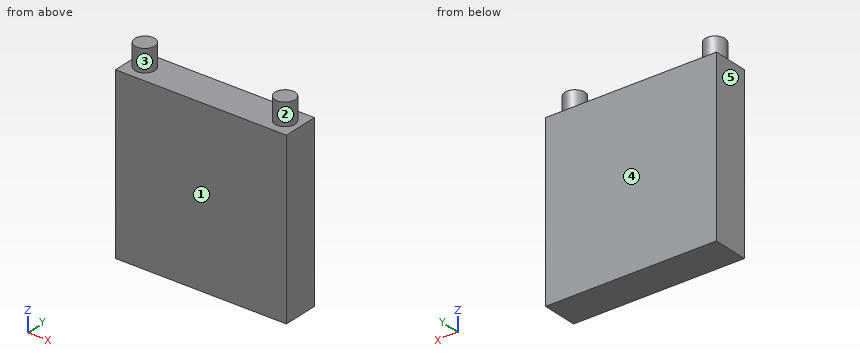
```python
from build123d import *

# Parameters (mm, degrees)
SKETCH_1_W      = 20
SKETCH_1_H      = 20
EXTRUDE_1_DEPTH = 4.2
SKETCH_2_R      = 1.173131764
EXTRUDE_2_DEPTH = 12.6


with BuildPart() as part:
    # 草图1 → 凸台-拉伸1 (new body)
    with BuildSketch(Plane(origin=(0, 0, 0), x_dir=(1, 0, 0), z_dir=(0, 1, 0))):
        Rectangle(SKETCH_1_W, SKETCH_1_H)
    extrude(amount=EXTRUDE_1_DEPTH)

    # 草图2 → 凸台-拉伸2 (add)
    with BuildSketch(Plane.XY):
        with Locations((-8.2, 2.1)):
            Circle(SKETCH_2_R)
        with Locations((8.2, 2.1)):
            Circle(SKETCH_2_R)
    extrude(amount=EXTRUDE_2_DEPTH)


solid = part.part
```
For this review, take the finished solid that the model builds, in its own axes (mm). Face numbers are marked on the shaded views. A direction names the side the tool comes from. Coordinates: 2 decimals unless noted, no trailing zeros. Write each loop counter-clockwise with the first axis right and the second up, starting at its lowest first coordinate (ties: lowest second). Pieces come first, ordered by that corner, then holes. Notation, with made-up numbers: (33, 46) -> (50, 46) arc R21 ccw to (50, 61) -> close; hole circle Ø5 at (-8, 76). An arc over 180 degrees is marked (long way). Put each result on its own line as item: value.
Q1. Take a section at D-D, the plane x = 3.75. State the section outline as (y, z) points, then the cut area to 3 significant figures.
From the geometry:
outline: (0, -10) -> (4.2, -10) -> (4.2, 10) -> (0, 10) -> close
area: 84.0 mm2
Q2. Wall thickness on L1, parallel to Z at x = -5.25, y = 1.1: over which ranges is the line inside the solid? List them lowest first.
From the geometry:
L1: z = -10 to 10
Q3. Take a section at C-C, the plane z = 11.25. State the section outline as (x, y) points.
From the geometry:
outline: circle Ø2.35 at (-8.2, 2.1); circle Ø2.35 at (8.2, 2.1)
Q4. Take a section at B-B, the plane x = 8.2. State the section outline as (y, z) points.
From the geometry:
outline: (0, -10) -> (4.2, -10) -> (4.2, 10) -> (3.27, 10) -> (3.27, 12.6) -> (0.93, 12.6) -> (0.93, 10) -> (0, 10) -> close
Q5. The part is to be moulded in two halves that separate along X. For the marked faces 3, 4 and 5, say which applies: +X half, -X half, draft (parallel to the pull), parting line (faces both ways), or undercut.
From the geometry:
face 3: undercut
face 4: draft
face 5: -X half
Q6. Tool access review of the marked faces 1 and 2: name each direction out of +Z, -Z, +X, -X, +Y, -Y from which nothing blocks a thin tool from reaching the whole face with its end or side.
From the geometry:
face 1: +Z, -Z, +X, -X, -Y
face 2: +Z
Q7. Take a section at A-A, the plane y = 2.1. State the section outline as (x, z) points.
From the geometry:
outline: (-10, -10) -> (10, -10) -> (10, 10) -> (9.37, 10) -> (9.37, 12.6) -> (7.03, 12.6) -> (7.03, 10) -> (-7.03, 10) -> (-7.03, 12.6) -> (-9.37, 12.6) -> (-9.37, 10) -> (-10, 10) -> close
Q8. Clearance check with a flat-ended pin moving along its axis: pin 1 Ø2 at (x, y) = (3, 1.5) entering from +Z. State where the tip first meets the part, or that it passes through.
From the geometry:
pin 1: stops at z = 10
